Verification items for the finished model (mm, model axes). A direction names the side the tool comes from. Give positions to 0.01 mm unless a question says otherwise; leave off trailing zeros. Answer in a Markdown table with one row per item.
```python
from build123d import *

# Parameters (mm, degrees)
MAIN_DEPTH        = 3.2
WHEEL_DEPTH       = 3.2
SKETCH3_W         = 25
SKETCH3_H         = 5
TABS_DEPTH        = 3.2
SCREW_HOLES_DEPTH = 3.2


with BuildPart() as part:
    # Sketch1 → main (new body)
    with BuildSketch(Plane(origin=(0, 0, 0), x_dir=(0, 0, -1), z_dir=(1, 0, 0))):
        with BuildLine():
            Line((-87.535437106, 0), (122.464562894, 0))
            Line((122.464562894, 0), (122.464562894, 30))
            add(Edge.make_bspline(
                [(-87.535437106, 20), (17.331032425, 30.296907598), (122.464562894, 30)],
                knots=[0, 0, 0, 1, 1, 1], degree=2))
            Line((-87.535437106, 20), (-87.535437106, 0))
        make_face()
    extrude(amount=MAIN_DEPTH)

    # Sketch2 → wheel (cut)
    with BuildSketch(Plane(origin=(3.2, 0, 0), x_dir=(0, 0, -1), z_dir=(1, 0, 0))):
        with BuildLine():
            Line((-87.535437106, 0), (-54.535437106, 0))
            Line((-54.535437106, 0), (-54.535437106, 4))
            ThreePointArc((-54.535437106, 4), (-57.464369294, 11.071067812), (-64.535437106, 14))
            Line((-64.535437106, 14), (-87.535437106, 14))
            Line((-87.535437106, 14), (-87.535437106, 0))
        make_face()
    extrude(amount=-WHEEL_DEPTH, mode=Mode.SUBTRACT)

    # Sketch3 → tabs (add)
    with BuildSketch(Plane(origin=(3.2, 0, 0), x_dir=(0, 0, -1), z_dir=(1, 0, 0))):
        with Locations((-25.035437106, -2.5)):
            Rectangle(SKETCH3_W, SKETCH3_H)
        with Locations((99.964562894, -2.5)):
            Rectangle(SKETCH3_W, SKETCH3_H)
    extrude(amount=-TABS_DEPTH)

    # Sketch5 → screw holes (cut)
    with BuildSketch(Plane(origin=(3.2, 0, 0), x_dir=(0, 0, -1), z_dir=(1, 0, 0))):
        Polygon((7.464562894, 0), (10.264562894, 0), (10.264562894, 9.7), (11.664562894, 9.7), (11.664562894, 12), (10.264562894, 12), (10.264562894, 17), (7.464562894, 17), (7.464562894, 12), (6.064562894, 12), (6.064562894, 9.7), (7.464562894, 9.7), align=None)
        Polygon((60.264562894, 0), (63.064562894, 0), (63.064562894, 9.7), (64.464562894, 9.7), (64.464562894, 12), (63.064562894, 12), (63.064562894, 17), (60.264562894, 17), (60.264562894, 12), (58.864562894, 12), (58.864562894, 9.7), (60.264562894, 9.7), align=None)
    extrude(amount=-SCREW_HOLES_DEPTH, mode=Mode.SUBTRACT)


solid = part.part
```
Q1. Draft check along Z on faces 5 (the face through (2, 14, -63.065)), 6 (the face through (0, 13, -16)), 7 (the face through (2, 15, -7.465)), 8 (the face through (1.622, 10.993, 57.387)). Enter one of: +Z half, -Z half, draft (parallel to the pull), parting line (faces both ways), or undercut.
Completed:
| item | result |
|---|---|
| face 5 | undercut |
| face 6 | draft |
| face 7 | undercut |
| face 8 | +Z half |
Q2. Tool access check on faces 1 (the face through (2, 14, 76)), 2 (the face through (3.2, 13, -16)), 3 (the face through (2, -3, -87.465)), 4 (the face through (2, 0, -117)). Record the directions out of +Z, -Z, +X, -X, +Y, -Y that give a thin tool (end or side, any length) a straight path to the whole face; none if there is none.
Completed:
| item | result |
|---|---|
| face 1 | +Z, +X, -X, -Y |
| face 2 | +Z, -Z, +X, +Y, -Y |
| face 3 | +X, -X, -Y |
| face 4 | -Z, +X, -X, -Y |
Q3. Thickness scan on line 1 (Z direction, x = 2.6, y = 1.5); line 2 (Y direction, x = 1.65, z = -106.5); line 3 (Z direction, x = 0.55, y = 8). Record the ranges inside material, lowest first.
Completed:
| item | result |
|---|---|
| line 1 | -122.46 to -63.06, -60.26 to -10.26, -7.46 to 54.54 |
| line 2 | -5 to 29.98 |
| line 3 | -122.46 to -63.06, -60.26 to -10.26, -7.46 to 55.37 |
Q4. Go/stop test with flat-tipped pins: P1, Ø1.2, axis at x = 1.5, y = 11, coming from the +Z side; P2, Ø1.5, axis at x = 0.5, z = -66, coming from the -Y side; P3, Ø1.4, axis at x = 1.5, z = -9.5, coming from the -Y side. Record where each tip stops, or that it passes through.
Completed:
| item | result |
|---|---|
| P1 | z = 58.04 |
| P2 | y = 0 |
| P3 | y = 17 |
